The model under review builds one solid part; all positions refer to its coordinate system, in mm. Face numbers are marked on the shaded views. A direction names the side the tool comes from. Give positions to 0.01 mm unless a question says otherwise; leave off trailing zeros. Write each loop counter-clockwise with the first axis right and the second up, starting at its lowest first coordinate (ties: lowest second). Pieces come first, ordered by that corner, then holes.
from build123d import *

# Parameters (mm, degrees)
SKETCH1_W                     = 8.5
SKETCH1_H                     = 11.5
BOSS_EXTRUDE1_DEPTH           = 3.5
SKETCH2_W                     = 6.5
SKETCH2_H                     = 9.5
CUT_EXTRUDE1_DEPTH            = 2.5
SKETCH3_R                     = 1.5
CUT_EXTRUDE2_DEPTH            = 8.574628704
SKETCH6_R                     = 0.5953125
CUT_EXTRUDE5_DEPTH            = 2.5
SKETCH7_R                     = 0.79375
CUT_EXTRUDE6_DEPTH            = 8.574628704
BOSS_EXTRUDE2_DEPTH           = 3.5
SKETCH14_W                    = 5.965258944
SKETCH14_H                    = 5.132960456
CUT_EXTRUDE8_DEPTH            = 0.75
TAP_DRILL_FOR_0_80_TAP1_D     = 1.19126
TAP_DRILL_FOR_0_80_TAP1_DEPTH = 7.11
TAP_DRILL_FOR_0_80_TAP1_TIP   = 0.357890611
CUT_EXTRUDE7_REACH            = 11.006
FILLET5_R                     = 1
FILLET6_R                     = 0.396875


with BuildPart() as part:
    # Sketch1 → Boss-Extrude1 (new body)
    with BuildSketch(Plane(origin=(0, 0, 0), x_dir=(1, 0, 0), z_dir=(0, 1, 0))):
        Rectangle(SKETCH1_W, SKETCH1_H)
    extrude(amount=BOSS_EXTRUDE1_DEPTH)

    # Sketch2 → Cut-Extrude1 (cut)
    with BuildSketch(Plane(origin=(0, 3.5, 0), x_dir=(1, 0, 0), z_dir=(0, 1, 0))):
        Rectangle(SKETCH2_W, SKETCH2_H)
    extrude(amount=-CUT_EXTRUDE1_DEPTH, mode=Mode.SUBTRACT)

    # Sketch3 → Cut-Extrude2 (cut, through all)
    with BuildSketch(Plane(origin=(0, 1, 0), x_dir=(1, 0, 0), z_dir=(0, 1, 0))):
        with Locations(Location((0.25, -1.75, 0), (0, 0, 270))):
            Circle(SKETCH3_R)
    extrude(amount=-CUT_EXTRUDE2_DEPTH, mode=Mode.SUBTRACT)

    # Sketch6 → Cut-Extrude5 (cut)
    with BuildSketch(Plane(origin=(0, 3.5, 0), x_dir=(1, 0, 0), z_dir=(0, 1, 0))):
        with Locations((2.829050494, -4.329050494)):
            Circle(SKETCH6_R)
    extrude(amount=-CUT_EXTRUDE5_DEPTH, mode=Mode.SUBTRACT)

    # Sketch7 → Cut-Extrude6 (cut, through all)
    with BuildSketch(Plane(origin=(0, 1, 0), x_dir=(1, 0, 0), z_dir=(0, 1, 0))):
        with Locations(Location((0.25, 1.25, 0), (0, 0, 270))):
            Circle(SKETCH7_R)
        with Locations(Location((-1.625, -3.5, 0), (0, 0, 270))):
            Circle(SKETCH7_R)
        with Locations(Location((2.125, -3.5, 0), (0, 0, 270))):
            Circle(SKETCH7_R)
    extrude(amount=-CUT_EXTRUDE6_DEPTH, mode=Mode.SUBTRACT)

    # Sketch9 → Boss-Extrude2 (add)
    with BuildSketch(Plane(origin=(0, 3.5, 0), x_dir=(1, 0, 0), z_dir=(0, 1, 0))):
        Polygon((-2.69064642, 6.789569053), (-4.770772156, 5.402818562), (-4.001541387, 4.248972409), (-3.411634369, 4.642243754), (-2.511322669, 5.242451554), (-1.921415651, 5.635722899), align=None)
    extrude(amount=-BOSS_EXTRUDE2_DEPTH)

    # Sketch14 → Cut-Extrude8 (cut)
    with BuildSketch(Plane(origin=(0, 3.5, 0), x_dir=(1, 0, 0), z_dir=(0, 1, 0))):
        with Locations((-3.25, 4.75)):
            Rectangle(SKETCH14_W, SKETCH14_H)
    extrude(amount=-CUT_EXTRUDE8_DEPTH, mode=Mode.SUBTRACT)

    # Tap Drill for #0-80 Tap1
    with Locations(Plane(origin=(-3.961538462, 0, -5.942307692), x_dir=(-0.8320502943378434, 0, 0.5547001962252295), z_dir=(-0.5547001962252295, 0, -0.8320502943378434))):
        with Locations((-0.27742214, 1.875)):
            Hole(TAP_DRILL_FOR_0_80_TAP1_D / 2, depth=TAP_DRILL_FOR_0_80_TAP1_DEPTH)
            with Locations((0, 0, -(TAP_DRILL_FOR_0_80_TAP1_DEPTH + TAP_DRILL_FOR_0_80_TAP1_TIP / 2))):  # 118° drill point
                Cone(0, TAP_DRILL_FOR_0_80_TAP1_D / 2, TAP_DRILL_FOR_0_80_TAP1_TIP, mode=Mode.SUBTRACT)

    # Sketch13 → Cut-Extrude7 (cut, up to next)
    with BuildSketch(Plane(origin=(0, 3.5, 0), x_dir=(1, 0, 0), z_dir=(0, 1, 0)), mode=Mode.PRIVATE) as cut_extrude7_sk1:
        Polygon((-1.997600385, 5.75), (-1.997600385, 4.75), (3.25, 1.170806318), (4.25, 1.170806318), (4.25, 5.75), align=None)
    cut_extrude7_tool1 = extrude(cut_extrude7_sk1.sketch, amount=-CUT_EXTRUDE7_REACH, mode=Mode.PRIVATE) & part.part
    # Sketch13 → Cut-Extrude7 (cut, up to next)
    with BuildSketch(Plane(origin=(0, 3.5, 0), x_dir=(1, 0, 0), z_dir=(0, 1, 0)), mode=Mode.PRIVATE) as cut_extrude7_sk2:
        Polygon((-4.25, 4.621660328), (-3.25, 3.121660328), (-3.25, -5.75), (-4.25, -5.75), align=None)
    cut_extrude7_tool2 = extrude(cut_extrude7_sk2.sketch, amount=-CUT_EXTRUDE7_REACH, mode=Mode.PRIVATE) & part.part
    add(cut_extrude7_tool1.solids().sort_by_distance((1.797917, 3.5, -3.996239))[0], mode=Mode.SUBTRACT)
    add(cut_extrude7_tool2.solids().sort_by_distance((-3.762992, 3.5, 0.929426))[0], mode=Mode.SUBTRACT)

    # Fillet5
    fillet5_edges = [part.edges().sort_by_distance(p)[0] for p in [
        (3.25, 0.5, -1.170806318),
        (-1.997600385, 0.5, -4.75),
        (-3.25, 0.5, -3.121660328),
    ]]
    fillet(fillet5_edges, radius=FILLET5_R)

    # Fillet6
    fillet6_edges = [part.edges().sort_by_distance(p)[0] for p in [
        (-3.25, 1.195357051, -4.75),
        (-3.25, 2.554642949, -4.75),
    ]]
    fillet(fillet6_edges, radius=FILLET6_R)


solid = part.part
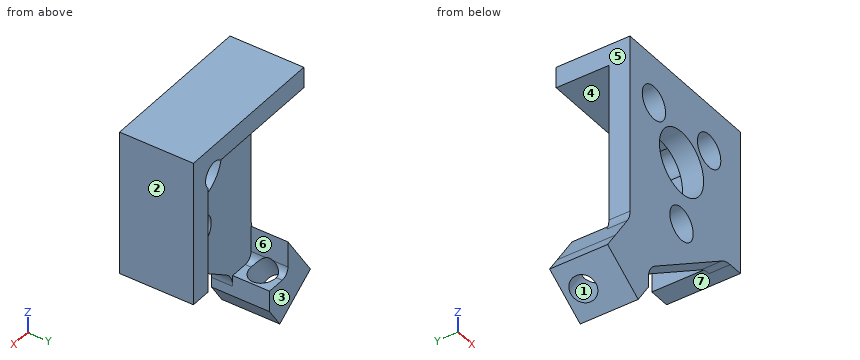
1) To check wall thickness, follow probe 1 along X at (y, z) = (0.75, 3.5); probe 2 along Z at (x, y) = (-1, 0.5); probe 3 along Z at (x, y) = (0.5, 2.9). State the ranges of each line that lie inside material, in increasing order.
2) Consider section B-B, the plane y = 2.2. Give the boundary of the cut face in (x, z).
3) Consider section C-C, the plane z = 1.75. Give the boundary of the cut face in (x, y).
4) Tool access review of the marked faces 4, 5, 6 and 7: name each direction out of +Z, -Z, +X, -X, +Y, -Y from which nothing blocks a thin tool from reaching the whole face with its end or side.
5) Consider section D-D, the plane x = 0. Give the boundary of the cut face in (y, z), then the cut area to 3 significant figures.
6) The part is to be moulded in two halves that separate along Y. For the marked faces 1, 2 and 3, say which applies: +Y half, -Y half, draft (parallel to the pull), parting line (faces both ways), or undercut.
7) Consider section A-A, the plane z = 3.5. Give the boundary of the cut face in (x, y), then the cut area to 4 significant figures.
8) Insertion check: pin 1 (0.8 mm diameter, centred on y = 1, z = -5.5, fed in from +X); pin 2 (0.5 mm diameter, centred on x = 3.5, y = 1, fed in from -Z); pin 3 (1.8 mm diameter, centred on x = 2.125, z = 3.5, fed in from +Y). Each pin has a flat end and moves straight along its axis. Give the tip position at first contact, or say it passes through.
Answer block:
1. probe 1: x = -3.25 to -2.42, -0.83 to 1.33, 2.92 to 4.25
1. probe 2: z = -4.07 to 0.92, 2.58 to 3.01, 3.99 to 5.75
1. probe 3: z = 4.75 to 5.75
2. outline: (-4.77, -5.4) - (-4.15, -5.82) - (-3.24, -4.46) arc R0.4 cw to (-3.25, -4.35) - (-3.25, -3.12) - close; (-3.32, -6.37) - (-2.69, -6.79) - (-2, -5.75) - (-2, -4.75) - (-2.23, -4.75) - close; (-3.25, 4.75) - (2.41, 4.75) arc R0.6 cw to (3.25, 3.91) - (3.25, -1.17) - (4.25, -1.17) - (4.25, 5.75) - (-3.25, 5.75) - close
3. outline: (-3.25, 0) - (-1.25, 0) - (-1.25, 1) - (-3.25, 1) - close; (1.75, 0) - (4.25, 0) - (4.25, 3.5) - (3.25, 3.5) - (3.25, 1) - (1.75, 1) - close
4. face 4: -X, +Y
4. face 5: +Z, -X, +Y, -Y
4. face 6: +X, +Y
4. face 7: -Z, +X, +Y
5. outline: (0, -3.39) - (1, -3.39) - (1, -2) - (0, -2) - close; (0, -0.5) - (1, -0.5) - (1, 0.27) - (0, 0.27) - close; (0, 3.23) - (1, 3.23) - (1, 4.75) - (3.5, 4.75) - (3.5, 5.75) - (0, 5.75) - close
5. area: 7.17 mm2
6. face 1: undercut
6. face 2: draft
6. face 3: +Y half
7. outline: (-3.25, 0) - (-2.42, 0) - (-2.42, 1) - (-3.25, 1) - close; (-0.83, 0) - (1.33, 0) - (1.33, 1) - (-0.83, 1) - close; (2.92, 0) - (4.25, 0) - (4.25, 3.5) - (3.25, 3.5) - (3.25, 1) - (2.92, 1) - close
7. area: 6.825 mm2
8. pin 1: stops at x = -1.98
8. pin 2: stops at z = -1.22
8. pin 3: stops at y = 1
